```python
from build123d import *

# Parameters (mm, degrees)
SKETCH1_W                                  = 96.6
SKETCH1_H                                  = 32
BOSS_EXTRUDE1_DEPTH                        = 3
SKETCH2_R                                  = 5
CUT_EXTRUDE1_DEPTH                         = 79.565348097
FRAISAGE_POUR_VIS_T_TE_FRAIS_E_BOM_2_COUNT = 2
FRAISAGE_POUR_VIS_T_TE_FRAIS_E_BOM_2_PITCH = 64.6


with BuildPart() as part:
    # Sketch1 → Boss-Extrude1 (new body)
    with BuildSketch(Plane.XY):
        with Locations((28.417538555, 0.671328671)):
            Rectangle(SKETCH1_W, SKETCH1_H)
    extrude(amount=BOSS_EXTRUDE1_DEPTH)

    # Sketch2 → Cut-Extrude1 (cut, through all)
    with BuildSketch(Plane.XY.offset(3)):
        with Locations((28.417538555, 0.671328671)):
            Circle(SKETCH2_R)
    extrude(amount=-CUT_EXTRUDE1_DEPTH, mode=Mode.SUBTRACT)

    # Esquisse3 → Fraisage pour vis à tête fraisée bombée #51 (revolve, cut)
    with BuildSketch(Plane(origin=(-3.882461445, 0.671328671, 3), x_dir=(0, -1, 0), z_dir=(1, 0, 0))):
        Polygon((0, 0), (0, 3), (2.54999998, 3), (2.54999998, 2.700000061), (5.250000041, 0), align=None)
    fraisage_pour_vis_t_te_frais_e_bomb_e = revolve(axis=Axis((-3.882461445, 0.671328671, 9.35), (0, 0, -1)), mode=Mode.SUBTRACT)

    # Fraisage pour vis _ t_te frais_e bom 2: Fraisage pour vis à tête fraisée bombée #51 ×2
    with Locations(*[(i * FRAISAGE_POUR_VIS_T_TE_FRAIS_E_BOM_2_PITCH, 0, 0) for i in range(1, FRAISAGE_POUR_VIS_T_TE_FRAIS_E_BOM_2_COUNT)]):
        add(fraisage_pour_vis_t_te_frais_e_bomb_e, mode=Mode.SUBTRACT)


solid = part.part
```
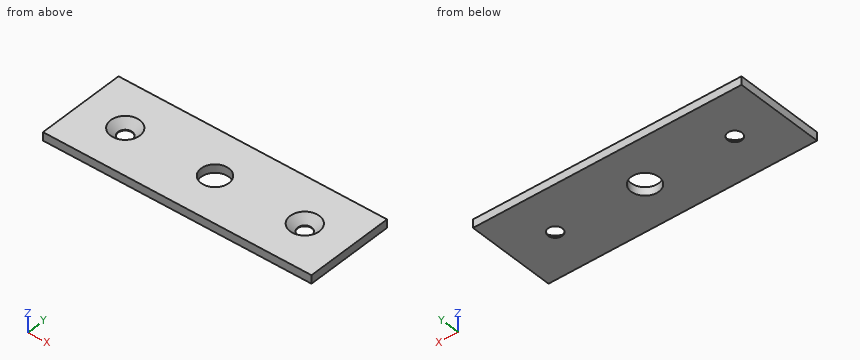
Verification items for the finished model (mm, model axes). Coordinates: 2 decimals unless noted, no trailing zeros. Order: outer loops, then holes, each group sorted by start corner. A loop starts at its lowest first (then second) coordinate and runs counter-clockwise, first axis right, second up. Notation, with made-up numbers: (10.5, 67.5) -> (31.5, 67.5) arc R17 cw to (31.5, 81.5) -> close; hole circle Ø10 at (69.5, -35.5). An arc over 180 degrees is marked (long way). Answer as CSV lines item,"result". Start each with the question number.
1) Cross-section at A-A, the plane z = 1.8. Record the boundary of the cut face in (x, y), then the cut area to 3 significant figures.
2) Cross-section at B-B, the plane x = 27. Record the boundary of the cut face in (y, z), then the cut area to 3 significant figures.
3) Gauge pin test, flat end, axial feed: pin 1 Ø4 at (x, y) = (64.5, -0.5) entering from +Z. Record the tip position at first contact, or that the pin passes through.
4) Material ranges on L1, parallel to X at y = 2.5, z = 2.6; L2, parallel to X at y = 1.5, z = 2.9; L3, parallel to Y at x = 26, z = 1.7, recorded low to high. Write a range as [from, to].
Conclusion:
1,outline,"(-19.88, -15.33) -> (76.72, -15.33) -> (76.72, 16.67) -> (-19.88, 16.67) -> close; hole circle Ø8.1 at (-3.88, 0.67); hole circle Ø10 at (28.42, 0.67); hole circle Ø8.1 at (60.72, 0.67)"
1,area,"2,910 mm²"
2,outline,"(-15.33, 0) -> (-4.12, 0) -> (-4.12, 3) -> (-15.33, 3) -> close; (5.47, 0) -> (16.67, 0) -> (16.67, 3) -> (5.47, 3) -> close"
2,area,"67.2 mm²"
3,pin 1,"stops at z = 3"
4,L1,"x = [-19.88, -8.37], [0.61, 23.76], [33.07, 56.23], [65.21, 76.72]"
4,L2,"x = [-19.88, -8.97], [1.2, 23.49], [33.35, 55.63], [65.8, 76.72]"
4,L3,"y = [-15.33, -3.71], [5.05, 16.67]"
